The model under review builds one solid part; all positions refer to its coordinate system, in mm. Face numbers are marked on the shaded views. A direction names the side the tool comes from. Round coordinates to 2 decimals unless told otherwise and drop trailing zeros. Order: outer loops, then holes, each group sorted by start corner. A loop starts at its lowest first (then second) coordinate and runs counter-clockwise, first axis right, second up.
1) Clearance check with flat-ended pins moving along their axes: P1, Ø6.5, axis at x = 11.5, z = 5.5, coming from the -Y side; P2, Ø1, axis at y = 19, z = 5.5, coming from the +X side; P3, Ø1.8, axis at x = 3, z = 6.5, coming from the -Y side; P4, Ø1.5, axis at x = 21, z = 10, coming from the -Y side. State where each tip first meets the part, or that it passes through.
2) Consider section B-B (z = 1). Give the boundary of the cut face in (x, y), then the cut area to 3 significant figures.
3) Machinability: for the marked faces 1, 2 and 3, which of the approach directions +Z, -Z, +X, -X, +Y, -Y give a long, thin tool a straight path to every point of the face, cutting with its end or side? Answer none if there is none.
4) Consider section A-A (x = 11.75). Give the boundary of the cut face in (y, z).
5) Consider section D-D (x = 27). Give the boundary of the cut face in (y, z), then the cut area to 3 significant figures.
6) To check wall thickness, follow L1, parallel to Z at x = 11.75, y = 18.7; L2, parallel to X at y = -2, z = 9; L3, parallel to Y at x = 31.5, z = 3.25. State the ranges of each line that lie inside material, in increasing order.
7) Consider section C-C (z = 5.5). Give the boundary of the cut face in (x, y).
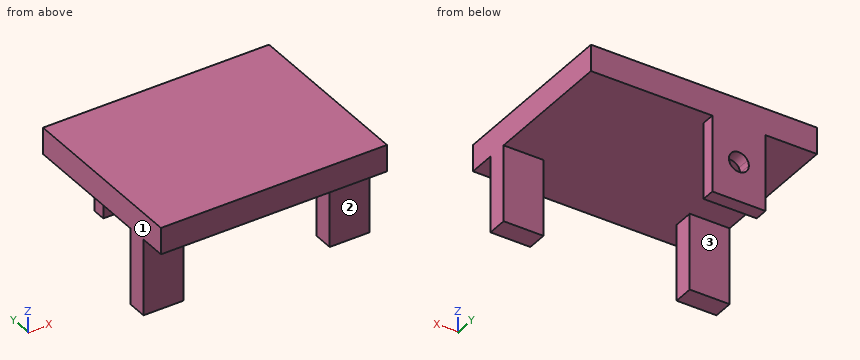
from build123d import *

# Parameters (mm, degrees)
F1_DEPTH = 3
F3_DEPTH = 4
F2_W     = 34
F2_H     = 4
F4_DEPTH = 23
F5_W     = 8
F5_H     = 11.5
F6_DEPTH = 2
F8_DEPTH = 2


with BuildPart() as f1:
    # F0 (on Front) → F1 (new body)
    with BuildSketch(Plane.XZ):
        Polygon((0, 15.5), (0, 0), (6, 0), (6, 11.5), (28, 11.5), (28, 0), (34, 0), (34, 15.5), align=None)
    extrude(amount=F1_DEPTH)

    # F2 (on face) → F3 (join)
    with BuildSketch(Plane.XZ.offset(3)):
        Polygon((0, 15.5), (0, 11.5), (6, 11.5), (28, 11.5), (34, 11.5), (34, 15.5), align=None)
    extrude(amount=F3_DEPTH)

    # F2 (on face) → F4 (join)
    with BuildSketch(Plane.XZ.offset(3)):
        with Locations((17, 13.5)):
            Rectangle(F2_W, F2_H)
    extrude(amount=-F4_DEPTH)

    # F5 (on face) → F6 (join)
    with BuildSketch(Plane(origin=(0, 20, 0), x_dir=(-1, 0, 0), z_dir=(0, 1, 0))):
        with Locations((-11.75, 5.75)):
            Rectangle(F5_W, F5_H)
    extrude(amount=-F6_DEPTH)

    # F7 (on face) → F8 (cut, through all)
    with BuildSketch(Plane(origin=(0, 20, 0), x_dir=(-1, 0, 0), z_dir=(0, 1, 0))):
        with BuildLine():
            ThreePointArc((-10.25, 5.93532), (-10.298761, 6.31467), (-10.441875, 6.669356))
            ThreePointArc((-10.441875, 6.669356), (-13.201239, 5.55597), (-10.25, 5.93532))
        make_face()
    extrude(amount=-F8_DEPTH, mode=Mode.SUBTRACT)


solid = f1.part
Answer below:
1. P1: stops at y = 18
1. P2: stops at x = 15.75
1. P3: stops at y = -3
1. P4: passes through
2. outline: (0, -3) - (6, -3) - (6, 0) - (0, 0) - close; (7.75, 18) - (15.75, 18) - (15.75, 20) - (7.75, 20) - close; (28, -3) - (34, -3) - (34, 0) - (28, 0) - close
2. area: 52.0 mm2
3. face 1: +Z, -Z, -X, +Y, -Y
3. face 2: -Z, +X, -X, -Y
3. face 3: -Z, +X, -X, +Y
4. outline: (-7, 11.5) - (18, 11.5) - (18, 7.44) - (20, 7.44) - (20, 15.5) - (-7, 15.5) - close; (18, 0) - (20, 0) - (20, 4.44) - (18, 4.44) - close
5. outline: (-7, 11.5) - (20, 11.5) - (20, 15.5) - (-7, 15.5) - close
5. area: 108 mm2
6. L1: z = 0 to 4.44, 7.44 to 15.5
6. L2: x = 0 to 6, 28 to 34
6. L3: y = -3 to 0
7. outline: (0, -3) - (6, -3) - (6, 0) - (0, 0) - close; (7.75, 18) - (10.31, 18) - (10.31, 20) - (7.75, 20) - close; (13.19, 18) - (15.75, 18) - (15.75, 20) - (13.19, 20) - close; (28, -3) - (34, -3) - (34, 0) - (28, 0) - close
